from build123d import *

# Parameters (mm, degrees)
SKETCH1_W            = 32
SKETCH1_H            = 32
BOSS_EXTRUDE1_DEPTH  = 7.36
SKETCH2_W            = 2.54
SKETCH2_H            = 19.05
BOSS_EXTRUDE2_DEPTH  = 6.5
SKETCH3_W            = 32
SKETCH3_H            = 32
BOSS_EXTRUDE3_DEPTH  = 1.5875
SKETCH4_R            = 1.5
CUT_EXTRUDE1_DEPTH   = 1.5875
LPATTERN1_COUNT      = 8
LPATTERN1_PITCH      = 3.97
LPATTERN1_COUNT_DIR2 = 8
LPATTERN1_PITCH_DIR2 = 3.97


with BuildPart() as part:
    # Sketch1 → Boss-Extrude1 (new body)
    with BuildSketch(Plane(origin=(0, 0, 0), x_dir=(1, 0, 0), z_dir=(0, 1, 0))):
        with Locations((16, 16)):
            Rectangle(SKETCH1_W, SKETCH1_H)
    extrude(amount=BOSS_EXTRUDE1_DEPTH)

    # Sketch2 → Boss-Extrude2 (add)
    with BuildSketch(Plane.XZ):
        with Locations((28.19, -16)):
            Rectangle(SKETCH2_W, SKETCH2_H)
        with Locations((3.81, -16)):
            Rectangle(SKETCH2_W, SKETCH2_H)
    extrude(amount=BOSS_EXTRUDE2_DEPTH)

    # Sketch3 → Boss-Extrude3 (add)
    with BuildSketch(Plane.XZ.offset(6.5)):
        with Locations((16, -16)):
            Rectangle(SKETCH3_W, SKETCH3_H)
    extrude(amount=BOSS_EXTRUDE3_DEPTH)

    # Sketch4 → Cut-Extrude1 (cut)
    with BuildSketch(Plane.XZ.offset(8.0875)):
        with Locations(Location((3.3, -28.7, 0), (0, 0, 270))):
            Circle(SKETCH4_R)
        with Locations(Location((28.7, -28.7, 0), (0, 0, 270))):
            Circle(SKETCH4_R)
        with Locations(Location((28.7, -3.3, 0), (0, 0, 270))):
            Circle(SKETCH4_R)
        with Locations(Location((3.3, -3.3, 0), (0, 0, 270))):
            Circle(SKETCH4_R)
    extrude(amount=-CUT_EXTRUDE1_DEPTH, mode=Mode.SUBTRACT)

    # Cut-Extrude2 cone 1 section (through the dimple's axis) → Cut-Extrude2 (revolve, cut)
    with BuildSketch(Plane(origin=(1.905, 7.36, -30.095), x_dir=(0, 0, 1), z_dir=(1, 0, 0))):
        Polygon((0, 0), (1.27, 0), (0, 0.223935265), align=None)
    cut_extrude2 = revolve(axis=Axis((1.905, 7.36, -30.095), (0, -1, 0)), mode=Mode.SUBTRACT)

    # LPattern1: Cut-Extrude2 8 × 8
    with Locations(*[(i * LPATTERN1_PITCH, 0, j * LPATTERN1_PITCH_DIR2) for i in range(LPATTERN1_COUNT) for j in range(LPATTERN1_COUNT_DIR2) if (i, j) != (0, 0)]):
        add(cut_extrude2, mode=Mode.SUBTRACT)


solid = part.part
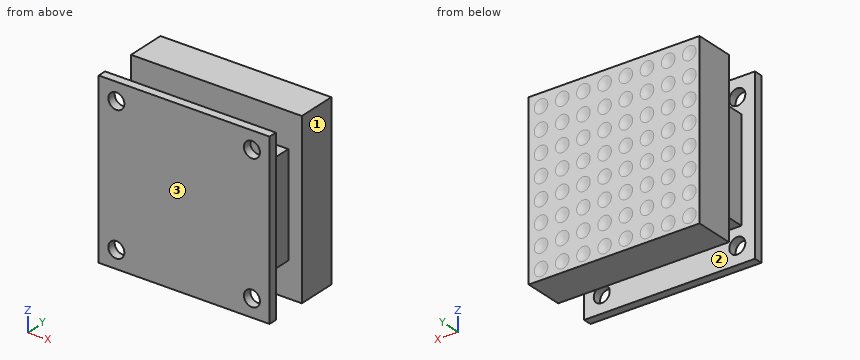
Here's how the part is built. I have some questions about the finished solid (model axes, mm). Face numbers are marked on the shaded views. Give positions to 0.01 mm unless a question says otherwise; leave off trailing zeros. Loops run counter-clockwise (first coordinate to the right, second up) from the corner with the lowest first, then second, coordinate; pieces in that order, holes last. Notation, with made-up numbers: (-23, 27) -> (-11, 27) arc R29 cw to (-11, 65) -> close; hole circle Ø5 at (-5, 40.5). An arc over 180 degrees is marked (long way). One line per item, written item: value.
Q1. I'm going to push flat-ended pins straight in: pin 1 Ø2 at (x, y) = (3.5, -2.5) entering from -Z (3 decimals); pin 2 Ø4 at (y, z) = (-4, -6) entering from -X; pin 3 Ø0.8 at (x, y) = (27.5, -2) entering from +Z (3 decimals). Where does each tip first touch, or does it pass through?
Answers follow:
pin 1: z = -25.525
pin 2: x = 2.54
pin 3: z = -6.475
Q2. Suppose I cut it at C-C on z = -16.5. Please give me the cut outline in (x, y), then the cut area to 3 significant figures.
Answers follow:
outline: (0, -8.09) -> (32, -8.09) -> (32, -6.5) -> (29.46, -6.5) -> (29.46, 0) -> (32, 0) -> (32, 7.36) -> (0, 7.36) -> (0, 0) -> (2.54, 0) -> (2.54, -6.5) -> (0, -6.5) -> close; hole (5.08, -6.5) -> (26.92, -6.5) -> (26.92, 0) -> (5.08, 0) -> close
area: 319 mm^2
Q3. Suppose I cut it at D-D on y = -7. Please give me the cut outline in (x, z).
Answers follow:
outline: (0, -32) -> (32, -32) -> (32, 0) -> (0, 0) -> close; hole circle Ø3 at (3.3, -28.7); hole circle Ø3 at (3.3, -3.3); hole circle Ø3 at (28.7, -28.7); hole circle Ø3 at (28.7, -3.3)
Q4. Suppose I cut it at B-B on y = -3.5. Please give me the cut outline in (x, z) (3 decimals).
Answers follow:
outline: (2.54, -25.525) -> (5.08, -25.525) -> (5.08, -6.475) -> (2.54, -6.475) -> close; (26.92, -25.525) -> (29.46, -25.525) -> (29.46, -6.475) -> (26.92, -6.475) -> close
Q5. If I drill on line 1 along X through (y, z) = (-7.3, -3.3); line 2 along Y through (x, z) = (26, -13); line 3 along X through (y, z) = (-5.5, -16), over which ranges is the centre line in solid material (lowest first)?
Answers follow:
line 1: 0 to 1.8, 4.8 to 27.2, 30.2 to 32
line 2: -8.09 to -6.5, 0 to 7.36
line 3: 2.54 to 5.08, 26.92 to 29.46
Q6. We'd pull the mould along Y, two halves only. Please class the marked faces 1, 2 and 3: pulls with the +Y half, pulls with the -Y half, needs draft (parallel to the pull), parting line crosses it, or undercut.
Answers follow:
face 1: needs draft
face 2: undercut
face 3: pulls with the -Y half
Q7. Suppose I cut it at A-A on x = 23.5. Please give me the cut outline in (y, z), then the cut area to 3 significant figures.
Answers follow:
outline: (-8.09, -32) -> (-6.5, -32) -> (-6.5, 0) -> (-8.09, 0) -> close; (0, -32) -> (7.36, -32) -> (7.36, 0) -> (0, 0) -> close
area: 286 mm^2
